Geometry: final body of the model. Coordinates: model frame, mm. Give positions to 0.01 mm unless a question says otherwise; leave off trailing zeros. Order: outer loops, then holes, each group sorted by start corner. A loop starts at its lowest first (then second) coordinate and runs counter-clockwise, first axis right, second up. Notation, with made-up numbers: (-35.75, 64) - (19.25, 64) arc R19 cw to (19.25, 71) - close; hole circle Ø11 at (-38, 2.25). An arc over 180 degrees is marked (long way). One line per item, written item: value.
Autodesk Inventor part; units mm, degrees
ref_plane "YZ Plane" through (0, 0, 0) normal (1, 0, 0) x (0, 1, 0)
ref_plane "XZ Plane" through (0, 0, 0) normal (0, 1, 0) x (-1, 0, 0)
ref_plane "XY Plane" through (0, 0, 0) normal (0, 0, 1) x (1, 0, 0)
sketch "Sketch1" plane through (0, 0, 0) normal (0, 0, 1) x (1, 0, 0)
  arc A0 (0, 6.35) -> (0, -6.35) centre (0, 0) ccw
  arc A1 (44.45, -6.35) -> (44.45, 6.35) centre (44.45, 0) ccw
  line L0 (0, -6.35) -> (44.45, -6.35)
  line L1 (44.45, 6.35) -> (0, 6.35)
  line L2 (-2.6416, -3.1496) -> (2.6416, -3.1496)
  line L3 (3.1496, -2.6416) -> (3.1496, 2.6416)
  line L4 (2.6416, 3.1496) -> (-2.6416, 3.1496)
  line L5 (-3.1496, 2.6416) -> (-3.1496, -2.6416)
  line L6 (-3.1496, -3.1496) -> (3.1496, 3.1496) construction
  line L7 (3.1496, -3.1496) -> (-3.1496, 3.1496) construction
  line L8 (41.8084, -3.1496) -> (47.0916, -3.1496)
  line L9 (47.5996, -2.6416) -> (47.5996, 2.6416)
  line L10 (47.0916, 3.1496) -> (41.8084, 3.1496)
  line L11 (41.3004, 2.6416) -> (41.3004, -2.6416)
  line L12 (41.3004, -3.1496) -> (47.5996, 3.1496) construction
  line L13 (47.5996, -3.1496) -> (41.3004, 3.1496) construction
  arc A2 (-2.6416, 3.1496) -> (-3.1496, 2.6416) centre (-2.6416, 2.6416) ccw
  arc A3 (3.1496, 2.6416) -> (2.6416, 3.1496) centre (2.6416, 2.6416) ccw
  arc A4 (2.6416, -3.1496) -> (3.1496, -2.6416) centre (2.6416, -2.6416) ccw
  arc A5 (-3.1496, -2.6416) -> (-2.6416, -3.1496) centre (-2.6416, -2.6416) ccw
  arc A6 (47.0916, -3.1496) -> (47.5996, -2.6416) centre (47.0916, -2.6416) ccw
  arc A7 (41.3004, -2.6416) -> (41.8084, -3.1496) centre (41.8084, -2.6416) ccw
  arc A8 (41.8084, 3.1496) -> (41.3004, 2.6416) centre (41.8084, 2.6416) ccw
  arc A9 (47.5996, 2.6416) -> (47.0916, 3.1496) centre (47.0916, 2.6416) ccw
  circle A10 centre (9.525, 0) radius 2.0955
  circle A11 centre (34.6456, 0) radius 2.0955
  dimension "d2" = 12.7
  dimension "d3" = 12.7
  dimension "d5" = 6.2992
  dimension "d6" = 6.2992
  dimension "d7" = 6.2992
  dimension "d8" = 6.2992
  dimension "d9" = 0.508
  dimension "d12" = 4.191
  dimension "d13" = 4.191
extrude "Extrusion1" add sketch "Sketch1" along normal blind 1.5875
properties part number "Gearbox Mirrored" material "Acetal Resin, White"
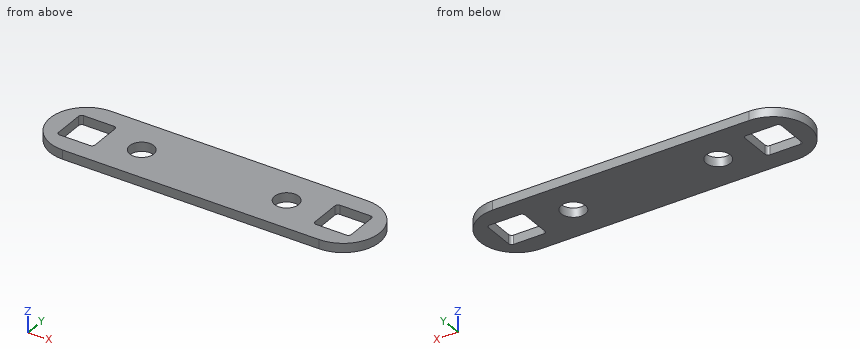
1) Section B-B, the plane y = 0. Return loops of the section in (x, z), then the cut area to 3 significant figures.
Answers below:
outline: (-6.35, 0) - (-3.15, 0) - (-3.15, 1.59) - (-6.35, 1.59) - close; (3.15, 0) - (7.43, 0) - (7.43, 1.59) - (3.15, 1.59) - close; (11.62, 0) - (32.55, 0) - (32.55, 1.59) - (11.62, 1.59) - close; (36.74, 0) - (41.3, 0) - (41.3, 1.59) - (36.74, 1.59) - close; (47.6, 0) - (50.8, 0) - (50.8, 1.59) - (47.6, 1.59) - close
area: 57.4 mm^2
2) Section D-D, the plane x = 8. Return loops of the section in (y, z), then the cut area to 3 significant figures.
Answers below:
outline: (-6.35, 0) - (-1.44, 0) - (-1.44, 1.59) - (-6.35, 1.59) - close; (1.44, 0) - (6.35, 0) - (6.35, 1.59) - (1.44, 1.59) - close
area: 15.6 mm^2
3) Section A-A, the plane x = 43.5. Return loops of the section in (y, z).
Answers below:
outline: (-6.35, 0) - (-3.15, 0) - (-3.15, 1.59) - (-6.35, 1.59) - close; (3.15, 0) - (6.35, 0) - (6.35, 1.59) - (3.15, 1.59) - close
4) First-contact query: pin 1 (0.5 mm diameter, centred on y = -1, z = 0.5, fed in from +X). Flat tip, straight axial feed; report the tip coordinate or a pass-through.
Answers below:
pin 1: x = 50.76
5) Section C-C, the plane z = 0.5. Count the separate pieces of the cut face and the enclosed holes in it, then the cut area to 3 significant figures.
Answers below:
separate pieces: 1
enclosed holes: 4
area: 585 mm^2
6) Material intervals for line 1 along X through (y, z) = (1, 1.1); line 2 along X through (y, z) = (-0.5, 0.1); line 3 along X through (y, z) = (-2.75, 0.75), sorted ascending.
Answers below:
line 1: -6.27 to -3.15, 3.15 to 7.68, 11.37 to 32.8, 36.49 to 41.3, 47.6 to 50.72
line 2: -6.33 to -3.15, 3.15 to 7.49, 11.56 to 32.61, 36.68 to 41.3, 47.6 to 50.78
line 3: -5.72 to -3.14, 3.14 to 41.31, 47.59 to 50.17
